Autodesk Inventor part; units mm, degrees
ref_plane "YZ Plane" through (0, 0, 0) normal (1, 0, 0) x (0, 1, 0)
ref_plane "XZ Plane" through (0, 0, 0) normal (0, 1, 0) x (-1, 0, 0)
ref_plane "XY Plane" through (0, 0, 0) normal (0, 0, 1) x (1, 0, 0)
sketch "Sketch1" plane through (0, 0, 0) normal (0, 0, 1) x (1, 0, 0)
  line L0 (-39.344, -1.4316) -> (-39.3671, -1.4316)
  line L1 (-39.344, -1.4316) -> (-52.044, -1.4316)
  line L2 (-39.344, -1.4316) -> (-45.694, -1.4316)
  line L3 (-39.344, -1.4316) -> (-46.964, -1.4316)
  line L4 (-46.964, -1.4316) -> (-46.964, -22.4724)
  line L5 (-46.964, -7.7816) -> (-59.664, -7.7816)
  line L6 (-59.664, -7.7816) -> (-59.664, -1.4316)
  arc A0 (-39.344, -1.4316) -> (30.4598, -1.4316) centre (-4.4421, -0.1616) ccw
  line L7 (30.4598, -1.4316) -> (43.1598, -1.4316)
  arc A1 (-46.964, -22.4724) -> (38.0798, -22.4724) centre (-4.4421, -0.1616) ccw
  line L8 (30.4598, -1.4316) -> (38.0798, -1.4316)
  line L9 (38.0798, -1.4316) -> (38.0798, -22.4724)
  line L10 (38.0798, -7.7816) -> (50.7798, -7.7816)
  line L11 (50.7798, -7.7816) -> (50.7798, -1.4316)
  line L12 (43.1598, -1.4316) -> (50.7798, -1.4316)
  line L13 (-52.044, -1.4316) -> (-59.664, -1.4316)
  line L14 (-46.964, -42.5386) -> (-46.964, -22.4724)
  line L15 (-46.964, -63.265) -> (-46.964, -42.5386)
  line L16 (-46.964, -22.4724) -> (-31.3118, -22.4724)
  line L17 (24.2345, -20.0969) -> (38.1472, -20.0969)
  line L18 (38.0798, -22.4724) -> (38.0798, -63.265)
  line L19 (38.0798, -63.265) -> (-46.964, -63.265)
  point P0 (0, 0)
  point P1 (0, 0)
  dimension "d0" = 69.85
  dimension "d1" = 12.7
  dimension "d2" = 12.7
  dimension "d3" = 7.62
  dimension "d4" = 7.62
  dimension "d5" = 7.62
  dimension "d6" = 7.62
  dimension "d7" = 6.35
  dimension "d8" = 6.35
  dimension "d17" = 61.8334
extrude "Extrusion1" add sketch "Sketch1" along normal blind 12.7
sketch "Sketch2" plane through (-59.664, -1.4316, 0) normal (0, 1, 0) x (1, 0, 0)
  circle A0 centre (7.62, -6.35) radius 4.064
  circle A1 centre (102.8238, -6.35) radius 4.064
  line L0 (90.1238, 0) -> (90.1238, -12.7)
  line L1 (20.32, 0) -> (20.32, -12.7)
  point P0 (59.664, 0)
  dimension "d11" = 12.7
  dimension "d12" = 12.7
  dimension "d13" = 8.128
  dimension "d14" = 8.128
extrude "Extrusion2" cut sketch "Sketch2" against normal blind 25.4
properties part number "REAL MOTOR MOUNT 2.75 TOP"
Build history of the part. All positions in model axes, mm. A direction names the side the tool comes from. Coordinates: 2 decimals unless noted, no trailing zeros. Write each loop counter-clockwise with the first axis right and the second up, starting at its lowest first coordinate (ties: lowest second). Pieces come first, ordered by that corner, then holes.
1. Drop flat-ended pins along their axis: pin 1 (6.5 mm diameter, centred on x = 42, z = 6, fed in from -Y); pin 2 (6.5 mm diameter, centred on x = 43.16, z = 6.35, fed in from +Y); pin 3 (2 mm diameter, centred on y = -53.5, z = 7, fed in from -X); pin 4 (1.5 mm diameter, centred on y = -14.5, z = 2, fed in from +X). Give the stop position or say it passes through.
Answer block:
pin 1: stops at y = -7.78
pin 2: passes through
pin 3: stops at x = -46.96
pin 4: stops at x = 38.08
2. 3-axis set-ups, long thin cutter, end or side, ignore diameter. For faces 5 (the flat face through (-46.964, -35, 6)), 6 (the flat face through (38.08, -35, 6)), 7 (the flat face through (50.78, -5, 6)): which of +Z, -Z, +X, -X, +Y, -Y reach the whole face in a straight line?
Answer block:
face 5: +Z, -Z, -X, -Y
face 6: +Z, -Z, +X, -Y
face 7: +Z, -Z, +X, +Y, -Y
3. Drill centre lines: probe 1 along X at (y, z) = (-3, 6.35); probe 2 along X at (y, z) = (-5.25, 6.35); probe 3 along Z at (x, y) = (43.5, -5.5). Where is each one in solid material? Low to high.
Answer block:
probe 1: x = -59.66 to -56.11, -47.98 to -39.25, 30.37 to 39.1, 47.22 to 50.78
probe 2: x = -59.66 to -56.11, -47.98 to -38.99, 30.11 to 39.1, 47.22 to 50.78
probe 3: z = 0 to 2.3, 10.4 to 12.7
4. Band-saw the part on D-D, the plane y = -45. Give the cut face in (x, z).
Answer block:
outline: (-46.96, 0) - (38.08, 0) - (38.08, 12.7) - (-46.96, 12.7) - close
5. Pull direction Z, two halves, no side cores. Call faces 1 (the flat face through (-47, -1.432, 6)), 2 (the flat face through (-5, -39, 0)), 3 (the flat face through (-5, -39, 12.7)), 4 (the cylindrical face through (-48.168, -4.562, 5.129)): released by +Z, released by -Z, zero draft, split by the parting line, or undercut.
Answer block:
face 1: zero draft
face 2: released by -Z
face 3: released by +Z
face 4: undercut
6. Band-saw the part on A-A, the plane z = 6.35. Give the cut face in (x, y) (3 decimals), and give its area (3 significant figures).
Answer block:
outline: (-59.664, -7.782) - (-56.108, -7.782) - (-56.108, -1.432) - (-59.664, -1.432) - close; (-47.98, -7.782) - (-46.964, -7.782) - (-46.964, -63.265) - (38.08, -63.265) - (38.08, -7.782) - (39.096, -7.782) - (39.096, -1.432) - (30.46, -1.432) arc R34.925 cw to (-39.344, -1.432) - (-47.98, -1.432) - close; (47.224, -7.782) - (50.78, -7.782) - (50.78, -1.432) - (47.224, -1.432) - close
area: 3,490 mm2
7. Band-saw the part on B-B, the plane y = -29. Give the cut face in (x, z).
Answer block:
outline: (-46.96, 0) - (-24.14, 0) - (-24.14, 12.7) - (-46.96, 12.7) - close; (15.26, 0) - (38.08, 0) - (38.08, 12.7) - (15.26, 12.7) - close
8. Band-saw the part on C-C, the plane y = -20.5. Give the cut face in (x, z), and give its area (3 significant figures).
Answer block:
outline: (-46.96, 0) - (-32.83, 0) - (-32.83, 12.7) - (-46.96, 12.7) - close; (23.95, 0) - (38.08, 0) - (38.08, 12.7) - (23.95, 12.7) - close
area: 359 mm2
